Autodesk Inventor part; units mm, degrees
ref_plane "YZ Plane" through (0, 0, 0) normal (1, 0, 0) x (0, 1, 0)
ref_plane "XZ Plane" through (0, 0, 0) normal (0, 1, 0) x (-1, 0, 0)
ref_plane "XY Plane" through (0, 0, 0) normal (0, 0, 1) x (1, 0, 0)
sketch "Esboço1" plane through (0, 0, 0) normal (0, 0, 1) x (1, 0, 0)
  line L0 (-121, -21) -> (121, -21)
  line L1 (121, -21) -> (121, 21)
  line L2 (121, 21) -> (-121, 21)
  line L3 (-121, 21) -> (-121, -21)
  line L4 (-121, -21) -> (121, 21) construction
  line L5 (121, -21) -> (-121, 21) construction
  point P0 (0, 0)
  dimension "d0" = 242
  dimension "d1" = 42
extrude "Extrusão1" add sketch "Esboço1" along normal blind 3
sketch "Esboço2" plane through (0, 0, 3) normal (0, 0, 1) x (1, 0, 0)
  line L0 (121, 21) -> (-121, 21)
  line L1 (-121, 21) -> (-79, 21)
  line L2 (-79, 21) -> (-79, -21)
  line L3 (-79, -21) -> (-121, -21)
  line L4 (-121, -21) -> (-121, 21)
  line L5 (-115.5, -15.5) -> (-84.5, -15.5)
  line L6 (-84.5, -15.5) -> (-84.5, 15.5)
  line L7 (-84.5, 15.5) -> (-115.5, 15.5)
  line L8 (-115.5, 15.5) -> (-115.5, -15.5)
  line L9 (-115.5, -15.5) -> (-84.5, 15.5) construction
  line L10 (-84.5, -15.5) -> (-115.5, 15.5) construction
  point P0 (0, 0)
  point P1 (-100, 0)
  point P2 (-100, 21)
  point P3 (-100, 15.5)
  point P4 (-121, 0)
  point P5 (-115.5, 0)
  dimension "d4" = 42
  dimension "d5" = 42
  dimension "d6" = 31
  dimension "d7" = 31
hole "Furo1" at (-115.5, 15.5, 3) at (-84.5, 15.5, 3) at (-84.5, -15.5, 3) at (-115.5, -15.5, 3) direction (0, 0, -1) diameter 3 end through all
hole "Furo2" at (-100, 0, 3) direction (0, 0, -1) diameter 23 end through all
mirror "Espelhamento1" about plane through (0, 0, 0) normal (1, 0, 0) of "Furo1", "Furo2"
sketch "Esboço3" plane through (0, 0, 3) normal (0, 0, 1) x (1, 0, 0)
  circle A0 centre (64, 10.5) radius 1.621
  circle A1 centre (64, -10.5) radius 1.621
  circle A2 centre (-64, 10.5) radius 1.621
  circle A3 centre (-64, -10.5) radius 1.621
  point P0 (0, 0)
hole "Furo3" at (64, -10.5, 3) at (64, 10.5, 3) at (-64, 10.5, 3) at (-64, -10.5, 3) direction (0, 0, -1) diameter 4 end through all
properties part number "chapa lateral"
Geometry check sheet. Reference: the model listing, model coordinates, mm. Give positions to 0.01 mm unless a question says otherwise; leave off trailing zeros. Write each loop counter-clockwise with the first axis right and the second up, starting at its lowest first coordinate (ties: lowest second). Pieces come first, ordered by that corner, then holes. Notation, with made-up numbers: (53, 83.5) -> (108, 83.5) arc R8 cw to (108, 89.5) -> close; hole circle Ø6 at (-31, 84). An arc over 180 degrees is marked (long way). Use one line per item in the form item = value.
Item 1: Mould release check, pull along X, two halves, no side actions. Record for faces 1 (the flat face through (-2, 0, 0)), 2 (the cylindrical face through (62.017, 10.76, 1.479)), 3 (the cylindrical face through (111.227, 2.493, 1.479)): released by +X, released by -X, zero draft, split by the parting line, or undercut.
Results list:
face_1 = zero draft
face_2 = undercut
face_3 = undercut
Item 2: Sectioned sample at D-D on y = -2. Enter the section's corners in (x, z).
Results list:
outline = (-121, 0) -> (-111.32, 0) -> (-111.32, 3) -> (-121, 3) -> close; (-88.68, 0) -> (88.68, 0) -> (88.68, 3) -> (-88.68, 3) -> close; (111.32, 0) -> (121, 0) -> (121, 3) -> (111.32, 3) -> close
Item 3: Depth check by flat-ended pin: pin 1 Ø5 at (x, y) = (-13, -9.5) entering from -Z. Enter the tip coordinate at first touch or a pass-through.
Results list:
pin_1 = 0
Item 4: Sectioned sample at A-A on x = -64. Enter the section's corners in (y, z).
Results list:
outline = (-21, 0) -> (-12.5, 0) -> (-12.5, 3) -> (-21, 3) -> close; (-8.5, 0) -> (8.5, 0) -> (8.5, 3) -> (-8.5, 3) -> close; (12.5, 0) -> (21, 0) -> (21, 3) -> (12.5, 3) -> close
Item 5: Sectioned sample at C-C on z = 1.05. Count the separate pieces of the cut face and the enclosed holes in it, plus the area to 3 significant figures.
Results list:
separate_pieces = 1
enclosed_holes = 14
area = 9,230 mm2
Item 6: Sectioned sample at B-B on x = 100. Enter the section's corners in (y, z).
Results list:
outline = (-21, 0) -> (-11.5, 0) -> (-11.5, 3) -> (-21, 3) -> close; (11.5, 0) -> (21, 0) -> (21, 3) -> (11.5, 3) -> close
Item 7: Scan lines: line 1 (Y direction, x = 115.5, z = 1.3); line 2 (X direction, y = 1, z = 1.3); line 3 (X direction, y = 15.5, z = 1.65). Record each from-to range of solid material in increasing order.
Results list:
line_1 = -21 to -17, -14 to 14, 17 to 21
line_2 = -121 to -111.46, -88.54 to 88.54, 111.46 to 121
line_3 = -121 to -117, -114 to -86, -83 to 83, 86 to 114, 117 to 121
